```python
from build123d import *

# Parameters (mm, degrees)
EXTRUDE_1_DEPTH     = 350
SKETCH_2_R          = 3
SKETCH_2_W          = 24
SKETCH_2_H          = 12.465583579
CUT_EXTRUDE_1_DEPTH = 350


with BuildPart() as part:
    # 草图1 → 凸台-拉伸1 (new body)
    with BuildSketch(Plane.XY):
        Polygon((-34.186090226, 5.411678692), (-33.186090226, 5.411678692), (-33.186090226, -5.088321308), (8.813909774, -5.088321308), (8.813909774, 5.411678692), (9.813909774, 5.411678692), (9.813909774, -6.088321308), (-34.186090226, -6.088321308), align=None)
    extrude(amount=EXTRUDE_1_DEPTH)

    # 草图2 → 切除-拉伸1 (cut)
    with BuildSketch(Plane.XZ.offset(6.088321308)):
        with Locations((-12.186090226, 261)):
            Circle(SKETCH_2_R)
        with Locations((-12.186090226, 197)):
            Circle(SKETCH_2_R)
        with Locations((-12.186090226, 101)):
            Circle(SKETCH_2_R)
        with Locations((-12.186090226, 37)):
            Circle(SKETCH_2_R)
        with BuildLine():
            Line((-22.436090226, 280), (-22.436090226, 252))
            ThreePointArc((-22.436090226, 252), (-21.850303788, 250.585786438), (-20.436090226, 250))
            Line((-20.436090226, 250), (-3.936090226, 250))
            ThreePointArc((-3.936090226, 250), (-2.521876663, 250.585786438), (-1.936090226, 252))
            Line((-1.936090226, 252), (-1.936090226, 280))
            ThreePointArc((-1.936090226, 280), (-3.936090226, 282), (-5.936090226, 280))
            Line((-5.936090226, 280), (-5.936090226, 256))
            ThreePointArc((-5.936090226, 256), (-6.521876663, 254.585786438), (-7.936090226, 254))
            Line((-7.936090226, 254), (-16.436090226, 254))
            ThreePointArc((-16.436090226, 254), (-17.850303788, 254.585786438), (-18.436090226, 256))
            Line((-18.436090226, 256), (-18.436090226, 280))
            ThreePointArc((-18.436090226, 280), (-20.436090226, 282), (-22.436090226, 280))
        make_face()
        with BuildLine():
            Line((-14.436090226, 279.5), (-14.436090226, 273.5))
            ThreePointArc((-14.436090226, 273.5), (-12.186090226, 271.25), (-9.936090226, 273.5))
            Line((-9.936090226, 273.5), (-9.936090226, 279.5))
            ThreePointArc((-9.936090226, 279.5), (-12.186090226, 281.75), (-14.436090226, 279.5))
        make_face()
        with BuildLine():
            Line((-5.936090226, 216), (-5.936090226, 192))
            ThreePointArc((-5.936090226, 192), (-6.521876663, 190.585786438), (-7.936090226, 190))
            Line((-7.936090226, 190), (-16.436090226, 190))
            ThreePointArc((-16.436090226, 190), (-17.850303788, 190.585786438), (-18.436090226, 192))
            Line((-18.436090226, 192), (-18.436090226, 216))
            ThreePointArc((-18.436090226, 216), (-20.436090226, 218), (-22.436090226, 216))
            Line((-22.436090226, 216), (-22.436090226, 188))
            ThreePointArc((-22.436090226, 188), (-21.850303788, 186.585786438), (-20.436090226, 186))
            Line((-20.436090226, 186), (-3.936090226, 186))
            ThreePointArc((-3.936090226, 186), (-2.521876663, 186.585786438), (-1.936090226, 188))
            Line((-1.936090226, 188), (-1.936090226, 216))
            ThreePointArc((-1.936090226, 216), (-3.936090226, 218), (-5.936090226, 216))
        make_face()
        with BuildLine():
            Line((-14.436090226, 216.5), (-14.436090226, 210.5))
            ThreePointArc((-14.436090226, 210.5), (-12.186090226, 208.25), (-9.936090226, 210.5))
            Line((-9.936090226, 210.5), (-9.936090226, 216.5))
            ThreePointArc((-9.936090226, 216.5), (-12.186090226, 218.75), (-14.436090226, 216.5))
        make_face()
        with BuildLine():
            Line((-20.436090226, 91), (-3.936090226, 91))
            ThreePointArc((-3.936090226, 91), (-2.521876663, 91.585786438), (-1.936090226, 93))
            Line((-1.936090226, 93), (-1.936090226, 121))
            ThreePointArc((-1.936090226, 121), (-3.936090226, 123), (-5.936090226, 121))
            Line((-5.936090226, 121), (-5.936090226, 97))
            ThreePointArc((-5.936090226, 97), (-6.521876663, 95.585786438), (-7.936090226, 95))
            Line((-7.936090226, 95), (-16.436090226, 95))
            ThreePointArc((-16.436090226, 95), (-17.850303788, 95.585786438), (-18.436090226, 97))
            Line((-18.436090226, 97), (-18.436090226, 121))
            ThreePointArc((-18.436090226, 121), (-20.436090226, 123), (-22.436090226, 121))
            Line((-22.436090226, 121), (-22.436090226, 93))
            ThreePointArc((-22.436090226, 93), (-21.850303788, 91.585786438), (-20.436090226, 91))
        make_face()
        with BuildLine():
            Line((-9.936090226, 120.5), (-9.936090226, 114.5))
            ThreePointArc((-9.936090226, 114.5), (-12.186090226, 112.25), (-14.436090226, 114.5))
            Line((-14.436090226, 114.5), (-14.436090226, 120.5))
            ThreePointArc((-14.436090226, 120.5), (-12.186090226, 122.75), (-9.936090226, 120.5))
        make_face()
        with BuildLine():
            Line((-20.436090226, 27), (-3.936090226, 27))
            ThreePointArc((-3.936090226, 27), (-2.521876663, 27.585786438), (-1.936090226, 29))
            Line((-1.936090226, 29), (-1.936090226, 57))
            ThreePointArc((-1.936090226, 57), (-3.936090226, 59), (-5.936090226, 57))
            Line((-5.936090226, 57), (-5.936090226, 33))
            ThreePointArc((-5.936090226, 33), (-6.521876663, 31.585786438), (-7.936090226, 31))
            Line((-7.936090226, 31), (-16.436090226, 31))
            ThreePointArc((-16.436090226, 31), (-17.850303788, 31.585786438), (-18.436090226, 33))
            Line((-18.436090226, 33), (-18.436090226, 57))
            ThreePointArc((-18.436090226, 57), (-20.436090226, 59), (-22.436090226, 57))
            Line((-22.436090226, 57), (-22.436090226, 29))
            ThreePointArc((-22.436090226, 29), (-21.850303788, 27.585786438), (-20.436090226, 27))
        make_face()
        with BuildLine():
            Line((-9.936090226, 56.5), (-9.936090226, 50.5))
            ThreePointArc((-9.936090226, 50.5), (-12.186090226, 48.25), (-14.436090226, 50.5))
            Line((-14.436090226, 50.5), (-14.436090226, 56.5))
            ThreePointArc((-14.436090226, 56.5), (-12.186090226, 58.75), (-9.936090226, 56.5))
        make_face()
        with BuildLine():
            Line((-14.186090226, 313), (-14.186090226, 308))
            ThreePointArc((-14.186090226, 308), (-12.186090226, 306), (-10.186090226, 308))
            Line((-10.186090226, 308), (-10.186090226, 313))
            ThreePointArc((-10.186090226, 313), (-12.186090226, 315), (-14.186090226, 313))
        make_face()
        with BuildLine():
            Line((-14.436090226, 144.5), (-14.436090226, 138.5))
            ThreePointArc((-14.436090226, 138.5), (-12.186090226, 136.25), (-9.936090226, 138.5))
            Line((-9.936090226, 138.5), (-9.936090226, 144.5))
            ThreePointArc((-9.936090226, 144.5), (-12.186090226, 146.75), (-14.436090226, 144.5))
        make_face()
        with Locations((-12.186090226, 343.767208211)):
            Rectangle(SKETCH_2_W, SKETCH_2_H)
    extrude(amount=-CUT_EXTRUDE_1_DEPTH, mode=Mode.SUBTRACT)


solid = part.part
```
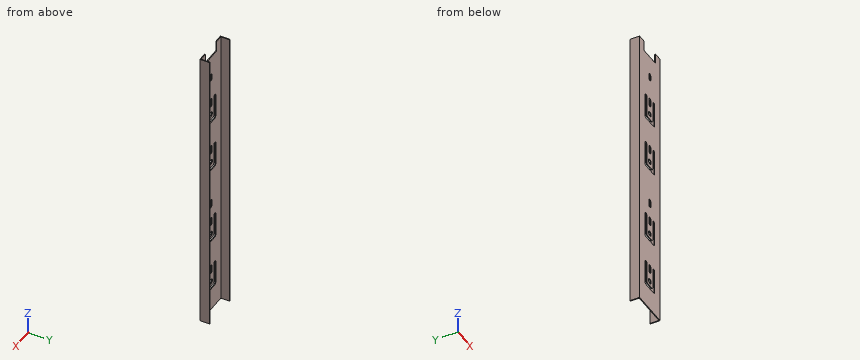
The listing builds one solid part. Answer for the finished solid, in the listing's coordinates (mm). Give positions to 0.01 mm unless a question says otherwise; leave off trailing zeros. Order: outer loops, then holes, each group sorted by start corner. A loop starts at its lowest first (then second) coordinate and runs counter-clockwise, first axis right, second up. Notation, with made-up numbers: (-7, -19) - (28, -19) arc R25 cw to (28, 10) - close; hole circle Ø11 at (54.5, 9). An arc over 180 degrees is marked (long way). Use one line per item in the form item = value. Start each with the question number.
(1) A cutting plane is placed at C-C, the plane z = 268. Write down the section's boundary in (x, y), then the cut area to 3 significant figures.
(2) A cutting plane is placed at B-B, the plane y = 3.5. Write down the section's boundary in (x, z), then the cut area to 3 significant figures.
(3) A flat-ended cylindrical pin translates along its axis: pin 1 Ø7 at (x, z) = (-12.19, 37) entering from +Y. Find the tip coordinate at first contact, or state that the pin passes through.
(4) A cutting plane is placed at A-A, the plane z = 37. Write down the section's boundary in (x, y).
(5) Consider line 1 (X direction, y = -5.5, z = 261); line 2 (X direction, y = 2.75, z = 173); line 3 (Y direction, x = 5.5, z = 23). Determine where each line is inside the solid, lowest interval first. Write a range as from..to.
Ans:
q1.outline = (-34.19, -6.09) - (-22.44, -6.09) - (-22.44, -5.09) - (-33.19, -5.09) - (-33.19, 5.41) - (-34.19, 5.41) - close; (-18.44, -6.09) - (-5.94, -6.09) - (-5.94, -5.09) - (-18.44, -5.09) - close; (-1.94, -6.09) - (9.81, -6.09) - (9.81, 5.41) - (8.81, 5.41) - (8.81, -5.09) - (-1.94, -5.09) - close
q1.area = 57.0 mm^2
q2.outline = (-34.19, 0) - (-33.19, 0) - (-33.19, 350) - (-34.19, 350) - close; (8.81, 0) - (9.81, 0) - (9.81, 350) - (8.81, 350) - close
q2.area = 700 mm^2
q3.pin_1 = -5.09
q4.outline = (-34.19, -6.09) - (-22.44, -6.09) - (-22.44, -5.09) - (-33.19, -5.09) - (-33.19, 5.41) - (-34.19, 5.41) - close; (-18.44, -6.09) - (-15.19, -6.09) - (-15.19, -5.09) - (-18.44, -5.09) - close; (-9.19, -6.09) - (-5.94, -6.09) - (-5.94, -5.09) - (-9.19, -5.09) - close; (-1.94, -6.09) - (9.81, -6.09) - (9.81, 5.41) - (8.81, 5.41) - (8.81, -5.09) - (-1.94, -5.09) - close
q5.line_1 = -34.19..-22.44, -18.44..-15.19, -9.19..-5.94, -1.94..9.81
q5.line_2 = -34.19..-33.19, 8.81..9.81
q5.line_3 = -6.09..-5.09
